CAD build for the part. Positions are in the model's coordinates, mm. A direction names the side the tool comes from. Round coordinates to 2 decimals unless told otherwise and drop trailing zeros. Order: outer loops, then holes, each group sorted by start corner. A loop starts at its lowest first (then second) coordinate and runs counter-clockwise, first axis right, second up. Notation, with made-up numbers: M 72,63.5 L 104,63.5 A19 ccw 104,67.5 Z; hole C -20,49.5 d9. An arc over 180 degrees is marked long. Put each result on its own line as item: value.
```python
from build123d import *

# Parameters (mm, degrees)
CUT_EXTRUDE1_DEPTH = 162.927340767
FILLET1_R          = 0.508


with BuildPart() as part:
    # Sketch1 → Revolve1 (revolve)
    with BuildSketch(Plane.XY, mode=Mode.PRIVATE) as revolve1_sk:
        Polygon((0, 161.544), (3.81, 161.544), (4.318, 153.924), (7.874, 153.924), (7.874, 124.46), (6.0579, 124.46), (6.0579, 0), (0, 0), align=None)
    revolve(revolve1_sk.sketch.rotate(Axis((0, 0, 0), (0, 1, 0)), 90), axis=Axis((0, 0, 0), (0, 1, 0)))

    # Sketch2 → Cut-Extrude1 (cut, through all)
    with BuildSketch(Plane.XY):
        with BuildLine():
            Line((-1.5875, 7.9375), (-1.5875, 10.8585))
            ThreePointArc((-1.5875, 10.8585), (0, 12.446), (1.5875, 10.8585))
            Line((1.5875, 10.8585), (1.5875, 7.9375))
            ThreePointArc((1.5875, 7.9375), (0, 6.35), (-1.5875, 7.9375))
        make_face()
    extrude(amount=-CUT_EXTRUDE1_DEPTH, mode=Mode.SUBTRACT)

    # Fillet1
    fillet1_edges = [part.edges().sort_by_distance(p)[0] for p in [
        (0, 153.924, 7.874),
        (0, 153.924, 4.318),
        (0, 161.544, 3.81),
    ]]
    fillet(fillet1_edges, radius=FILLET1_R)


solid = part.part
```
Item 1: Band-saw the part on B-B on y = 65. Give the cut face in (x, z), and give its area (3 significant figures).
Answers below:
outline: C 0,0 d12.12
area: 115 mm²
Item 2: Pin check, flat tips, straight feed: P1, Ø6, axis at y = 30.5, z = -1, coming from the +X side; P2, Ø3, axis at x = 0.5, z = 6, coming from the +Y side; P3, Ø3, axis at x = 0.5, y = 87.5, coming from the +Z side. Stop position of each tip, or through.
Answers below:
P1: x = 6.06
P2: y = 154
P3: z = 6.06
Item 3: Mould opens along X. For faces 4 (the flat face through (-1.588, 9, -3)), 5 (the flat face through (0, 153.924, 5)), 6 (the cylindrical face through (-0.035, 12.446, -2.987)), 7 (the conical face through (2.47, 157.69, 3.23)) say: pulls with the +X half, pulls with the -X half, needs draft (parallel to the pull), parting line crosses it, or undercut.
Answers below:
face 4: undercut
face 5: needs draft
face 6: undercut
face 7: parting line crosses it
Item 4: Band-saw the part on A-A on x = 0. Give the cut face in (y, z).
Answers below:
outline: M 0,-6.06 L 6.35,-6.06 L 6.35,0 L 12.45,0 L 12.45,-6.06 L 124.46,-6.06 L 124.46,-7.87 L 153.42,-7.87 A0.51 ccw 153.92,-7.37 L 153.92,-4.79 A0.51 cw 154.4,-4.29 L 161.07,-3.84 A0.51 ccw 161.54,-3.33 L 161.54,3.33 A0.51 ccw 161.07,3.84 L 154.4,4.29 A0.51 cw 153.92,4.79 L 153.92,7.37 A0.51 ccw 153.42,7.87 L 124.46,7.87 L 124.46,6.06 L 0,6.06 Z
Item 5: Probe line 1 along X through (y, z) = (135, 0.25); line 2 along Y through (x, z) = (5.75, 2); line 3 along Z through (x, y) = (-5, 130.5). List the from-to ranges inside material, lowest first. Write a range as [from, to].
Answers below:
line 1: [-7.87, 7.87]
line 2: [124.46, 153.92]
line 3: [-6.08, 6.08]
Item 6: Tool access for faces 1 (the flat face through (1.588, 9, -3)), 2 (the flat face through (0, 0, 0)), 3 (the cylindrical face through (5.914, 61.359, 1.313)): list every direction of +Z, -Z, +X, -X, +Y, -Y with a clear straight run to the whole face (end or side of a thin tool).
Answers below:
face 1: -Z
face 2: +Z, -Z, +X, -X, -Y
face 3: -Y
